Drawing for the job (mm, zero at the part's lowest x, y, z). A direction names the side the tool comes from. Round coordinates to 2 decimals unless told otherwise and drop trailing zeros. Write each loop counter-clockwise with the first axis right and the second up, starting at its lowest first coordinate (ties: lowest second). Pieces come first, ordered by that corner, then holes.
Item 1: Band-saw the part on B-B, the plane y = 14.25. Write the cut outline in (x, z).
Item 2: Drop a flat-ended pin along its axis: pin 1 Ø1.5 at (x, z) = (16.5, 11) entering from -Y. Give the stop position or say it passes through.
Item 3: Band-saw the part on C-C, the plane x = 8. Write the cut outline in (y, z), then the cut area to 3 significant figures.
Item 4: Wall check: probe 1 along X at (y, z) = (15.5, 10); probe 2 along X at (y, z) = (10, 10) (1 decimal); probe 3 along X at (y, z) = (3.5, 6) (1 decimal). Give the ranges that are in metal, low to high.
Item 5: 3-axis set-ups, long thin cutter, end or side, ignore diameter. For the marked faces 4, 5 and 6: which of +Z, -Z, +X, -X, +Y, -Y reach the whole face in a straight line?
Item 6: Band-saw the part on A-A, the plane x = 24. Write the cut outline in (y, z), then the cut area to 3 significant figures.
Item 7: Mould opens along Z. For the marked faces 1, 2 and 3 say: +Z half, -Z half, draft (parallel to the pull), parting line (faces both ways), or undercut.
Item 8: Band-saw the part on D-D, the plane z = 8.75. Count the separate pieces of the cut face and the enclosed holes in it, then the cut area to 3 significant figures.
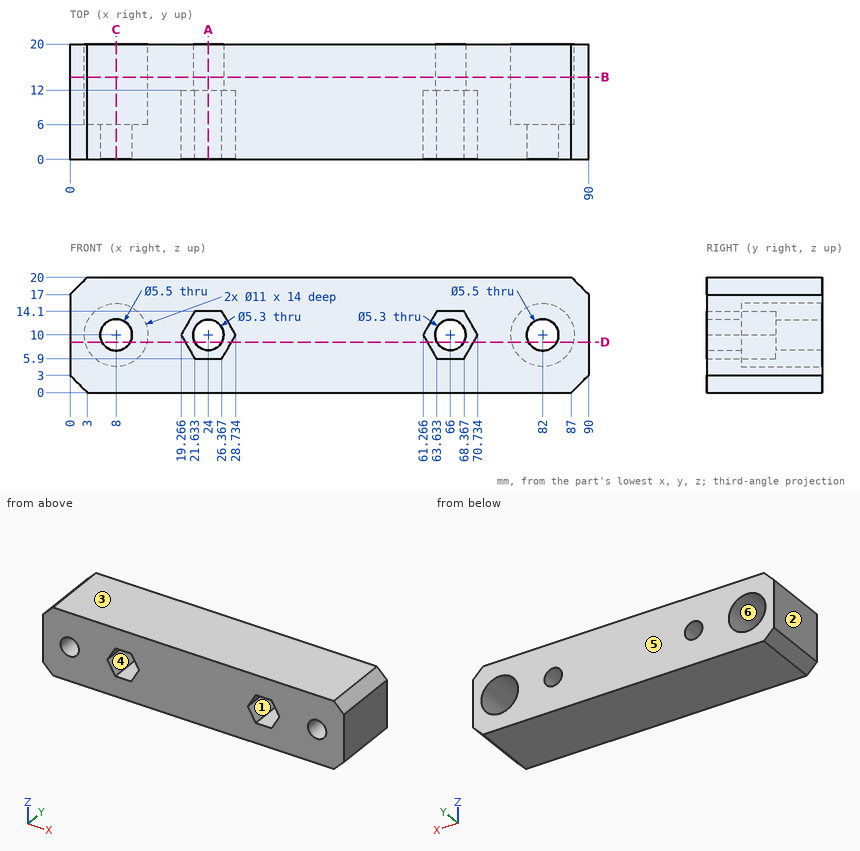
Results:
1. outline: (0, 3) - (3, 0) - (87, 0) - (90, 3) - (90, 17) - (87, 20) - (3, 20) - (0, 17) - close; hole circle Ø11 at (8, 10); hole circle Ø5.3 at (24, 10); hole circle Ø5.3 at (66, 10); hole circle Ø11 at (82, 10)
2. pin 1: stops at y = 0
3. outline: (0, 0) - (20, 0) - (20, 4.5) - (6, 4.5) - (6, 7.25) - (0, 7.25) - close; (0, 12.75) - (6, 12.75) - (6, 15.5) - (20, 15.5) - (20, 20) - (0, 20) - close
3. area: 213 mm2
4. probe 1: x = 0 to 2.5, 13.5 to 21.35, 26.65 to 63.35, 68.65 to 76.5, 87.5 to 90
4. probe 2: x = 0 to 2.5, 13.5 to 19.3, 28.7 to 61.3, 70.7 to 76.5, 87.5 to 90
4. probe 3: x = 0 to 21.6, 26.4 to 63.6, 68.4 to 90
5. face 4: -Y
5. face 5: +Z, -Z, +X, -X, +Y
5. face 6: +Y
6. outline: (0, 0) - (20, 0) - (20, 7.35) - (12, 7.35) - (12, 5.9) - (0, 5.9) - close; (0, 14.1) - (12, 14.1) - (12, 12.65) - (20, 12.65) - (20, 20) - (0, 20) - close
6. area: 259 mm2
7. face 1: undercut
7. face 2: draft
7. face 3: +Z half
8. separate pieces: 5
8. enclosed holes: 0
8. area: 1,170 mm2
